Verification items for the finished model (mm, model axes). Face numbers are marked on the shaded views. A direction names the side the tool comes from. Round coordinates to 2 decimals unless told otherwise and drop trailing zeros. Loops run counter-clockwise (first coordinate to the right, second up) from the corner with the lowest first, then second, coordinate; pieces in that order, holes last. Notation, with made-up numbers: (63.25, -31) -> (100.25, -31) arc R25 ccw to (100.25, -12) -> close; hole circle Ø6 at (-5.75, 81.25). An arc over 180 degrees is marked (long way). Use a Markdown table: item, result. Add a question column.
```python
from build123d import *

# Parameters (mm, degrees)
BOSS_EXTRUDE1_DEPTH       = 5
BOSS_EXTRUDE1_DEPTH_BACK  = 5
SKETCH1_R                 = 20.25
SKETCH1_R_2               = 13
SKETCH2_R                 = 13
SKETCH2_R_2               = 11.5
BOSS_EXTRUDE2_DEPTH       = 2
M5X0_8_TAPPED_HOLE1_D     = 4.2
M5X0_8_TAPPED_HOLE1_DEPTH = 15
M5X0_8_TAPPED_HOLE1_TIP   = 1.2618073
FILLET1_R                 = 2.5


with BuildPart() as part:
    # Sketch1 → Boss-Extrude1 (new, two sides: drawn at the far end of the back side and taken through both)
    # profile 1 of 3: a face of its own
    with BuildSketch(Plane.XY.offset(-BOSS_EXTRUDE1_DEPTH_BACK)):
        Circle(SKETCH1_R)
        Circle(SKETCH1_R_2, mode=Mode.SUBTRACT)
    # profile 2 of 3: a face of its own
    with BuildSketch(Plane.XY.offset(-BOSS_EXTRUDE1_DEPTH_BACK)):
        with BuildLine():
            Line((20.25, -44.75), (20.25, 0))
            ThreePointArc((20.25, 0), (14.318912319, -14.318912319), (0, -20.25))
            Line((0, -20.25), (10.25, -20.25))
            Line((10.25, -20.25), (10.25, -44.75))
            Line((10.25, -44.75), (20.25, -44.75))
        make_face()
    # profile 3 of 3: a face of its own
    with BuildSketch(Plane.XY.offset(-BOSS_EXTRUDE1_DEPTH_BACK)):
        with BuildLine():
            ThreePointArc((0, -20.25), (-14.318912319, -14.318912319), (-20.25, 0))
            Line((-20.25, 0), (-20.25, -44.75))
            Line((-20.25, -44.75), (-10.25, -44.75))
            Line((-10.25, -44.75), (-10.25, -20.25))
            Line((-10.25, -20.25), (0, -20.25))
        make_face()
    extrude(amount=BOSS_EXTRUDE1_DEPTH + BOSS_EXTRUDE1_DEPTH_BACK)

    # Sketch2 → Boss-Extrude2 (add)
    with BuildSketch(Plane(origin=(0, 0, -5), x_dir=(-1, 0, 0), z_dir=(0, 0, -1))):
        with Locations(Location((0, 0, 0), (0, 0, 180))):
            Circle(SKETCH2_R)
        Circle(SKETCH2_R_2, mode=Mode.SUBTRACT)
    extrude(amount=-BOSS_EXTRUDE2_DEPTH)

    # M5x0.8 Tapped Hole1
    with Locations(Plane(origin=(0, -44.75, 0), x_dir=(-1, 0, 0), z_dir=(0, -1, 0))):
        with Locations((15.75, 0), (-15.75, 0)):
            Hole(M5X0_8_TAPPED_HOLE1_D / 2, depth=M5X0_8_TAPPED_HOLE1_DEPTH)
            with Locations((0, 0, -(M5X0_8_TAPPED_HOLE1_DEPTH + M5X0_8_TAPPED_HOLE1_TIP / 2))):  # 118° drill point
                Cone(0, M5X0_8_TAPPED_HOLE1_D / 2, M5X0_8_TAPPED_HOLE1_TIP, mode=Mode.SUBTRACT)

    # Fillet1
    fillet1_edges = [part.edges().sort_by_distance(p)[0] for p in [
        (10.25, -20.25, 0),
        (-10.25, -20.25, 0),
    ]]
    fillet(fillet1_edges, radius=FILLET1_R)


solid = part.part
```
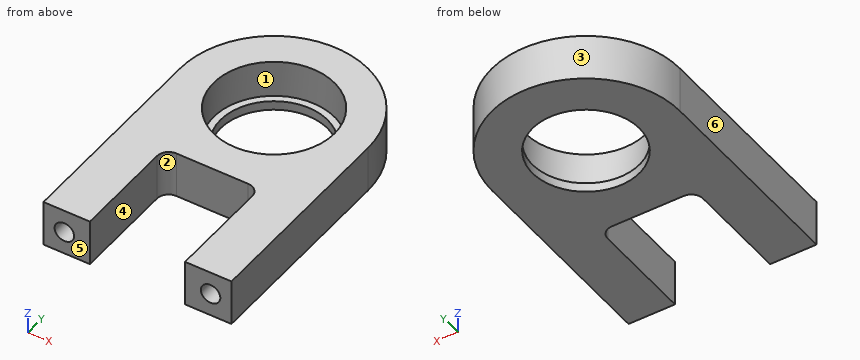
1) Access from +Z, -Z, +X, -X, +Y, -Y to the whole of each face (thin tool, end or side, straight path). Record for the marked faces 1, 2 and 3.
2) Thickness scan on line 1 (Y direction, x = 0, z = -3.5); line 2 (Z direction, x = 15.75, y = -33.25); line 3 (Y direction, x = 6, z = 1.5). Record the ranges inside material, lowest first.
3) Go/stop test with flat-tipped pins: pin 1 (5 mm diameter, centred on x = 7.5, z = -1, fed in from -Y); pin 2 (2.5 mm diameter, centred on x = 15.75, z = 0, fed in from +Y); pin 3 (20.5 mm diameter, centred on x = 0, y = 0, fed in from +Z); pin 4 (2 mm diameter, centred on x = 1.5, z = -1, fed in from +Y). Record where each tip stops, or that it passes through.
4) Release check for a two-part mould opening along X. For the marked faces 4, 5 and 6 record: released by +X, released by -X, zero draft, split by the parting line, or undercut.
5) Sectioned sample at D-D on y = -5. Enter the section's corners in (x, z).
6) Sectioned sample at A-A on y = -32. Enter the section's corners in (x, z), then the cut area to 3 significant figures.
7) Sectioned sample at B-B on x = 0. Enter the section's corners in (y, z).
8) Sectioned sample at C-C on y = -25.5. Enter the section's corners in (x, z).
Geometry results:
| question | item | result |
|---|---|---|
| 1 | face 1 | +Z |
| 1 | face 2 | +Z, -Z, -Y |
| 1 | face 3 | +Z, -Z, +Y |
| 2 | line 1 | -20.25 to -11.5, 11.5 to 20.25 |
| 2 | line 2 | -5 to -2.1, 2.1 to 5 |
| 2 | line 3 | -20.25 to -11.53, 11.53 to 19.34 |
| 3 | pin 1 | y = -21.66 |
| 3 | pin 2 | y = 14.14 |
| 3 | pin 3 | through |
| 3 | pin 4 | y = 20.24 |
| 4 | face 4 | undercut |
| 4 | face 5 | zero draft |
| 4 | face 6 | released by -X |
| 5 | outline | (-20.25, -5) -> (-10.36, -5) -> (-10.36, -3) -> (-12, -3) -> (-12, 5) -> (-20.25, 5) -> close; (10.36, -5) -> (20.25, -5) -> (20.25, 5) -> (12, 5) -> (12, -3) -> (10.36, -3) -> close |
| 6 | outline | (-20.25, -5) -> (-10.25, -5) -> (-10.25, 5) -> (-20.25, 5) -> close; (10.25, -5) -> (20.25, -5) -> (20.25, 5) -> (10.25, 5) -> close; hole circle Ø4.2 at (-15.75, 0); hole circle Ø4.2 at (15.75, 0) |
| 6 | area | 172 mm^2 |
| 7 | outline | (-20.25, -5) -> (-11.5, -5) -> (-11.5, -3) -> (-13, -3) -> (-13, 5) -> (-20.25, 5) -> close; (11.5, -5) -> (20.25, -5) -> (20.25, 5) -> (13, 5) -> (13, -3) -> (11.5, -3) -> close |
| 8 | outline | (-20.25, -5) -> (-10.25, -5) -> (-10.25, 5) -> (-20.25, 5) -> close; (10.25, -5) -> (20.25, -5) -> (20.25, 5) -> (10.25, 5) -> close |
